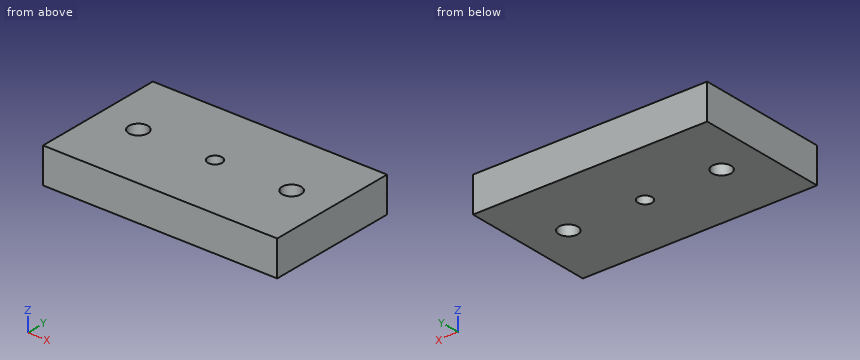
```python
from build123d import *

# Parameters (mm, degrees)
SKETCH1_W             = 40
SKETCH1_H             = 22.7
BOSS_EXTRUDE1_DEPTH   = 6
F_4_CLEARANCE_HOLE1_D = 3.2639
F_2_CLEARANCE_HOLE1_D = 2.4384


with BuildPart() as part:
    # Sketch1 → Boss-Extrude1 (new body)
    with BuildSketch(Plane.XY):
        Rectangle(SKETCH1_W, SKETCH1_H)
    extrude(amount=-BOSS_EXTRUDE1_DEPTH)

    # #4 Clearance Hole1 (through all)
    with Locations(Plane.XY):
        with Locations((-13.09, 0), (13.09, 0)):
            Hole(F_4_CLEARANCE_HOLE1_D / 2)

    # #2 Clearance Hole1 (through all)
    with Locations(Plane.XY):
        with Locations((0, 0)):
            Hole(F_2_CLEARANCE_HOLE1_D / 2)


solid = part.part
```
Check sheet for the modelled part. Datum: model origin and axes. Units: mm. Round coordinates to 2 decimals unless told otherwise and drop trailing zeros. Loops run counter-clockwise (first coordinate to the right, second up) from the corner with the lowest first, then second, coordinate; pieces in that order, holes last. Notation, with made-up numbers: (-28, 48.25) - (4, 48.25) arc R35 cw to (4, 82.25) - close; hole circle Ø2 at (-1.75, -9). An arc over 180 degrees is marked (long way). Answer as a JSON object with one key per item and string values. Group by question number.
Q1. Scan lines: line 1 along Y through (x, z) = (13.09, -1.8); line 2 along X through (y, z) = (-0.75, -0.4); line 3 along X through (y, z) = (1.25, -1.75). Record each from-to range of solid material in increasing order. Write a range as [from, to].
Q2. Sectioned sample at C-C, the plane z = -1.1. Enter the section's corners in (x, y).
Q3. Gauge pin test, flat ends, axial feed: P1, Ø2, axis at x = -13.09, y = 0, coming from the -Z side; P2, Ø5, axis at x = 13.09, y = 0, coming from the -Z side. Record the tip position at first contact, or that the pin passes through.
Q4. Sectioned sample at A-A, the plane x = -13.09. Enter the section's corners in (y, z).
Q5. Sectioned sample at B-B, the plane y = 0. Enter the section's corners in (x, z), plus the area to 3 significant figures.
Q6. Sectioned sample at D-D, the plane x = 0. Enter the section's corners in (y, z).
Solution:
{
 "1": {"line 1": "y = [-11.35, -1.63], [1.63, 11.35]", "line 2": "x = [-20, -14.54], [-11.64, -0.96], [0.96, 11.64], [14.54, 20]", "line 3": "x = [-20, -14.14], [-12.04, 12.04], [14.14, 20]"},
 "2": {"outline": "(-20, -11.35) - (20, -11.35) - (20, 11.35) - (-20, 11.35) - close; hole circle Ø3.26 at (-13.09, 0); hole circle Ø2.44 at (0, 0); hole circle Ø3.26 at (13.09, 0)"},
 "3": {"P1": "passes through", "P2": "stops at z = -6"},
 "4": {"outline": "(-11.35, -6) - (-1.63, -6) - (-1.63, 0) - (-11.35, 0) - close; (1.63, -6) - (11.35, -6) - (11.35, 0) - (1.63, 0) - close"},
 "5": {"outline": "(-20, -6) - (-14.72, -6) - (-14.72, 0) - (-20, 0) - close; (-11.46, -6) - (-1.22, -6) - (-1.22, 0) - (-11.46, 0) - close; (1.22, -6) - (11.46, -6) - (11.46, 0) - (1.22, 0) - close; (14.72, -6) - (20, -6) - (20, 0) - (14.72, 0) - close", "area": "186 mm²"},
 "6": {"outline": "(-11.35, -6) - (-1.22, -6) - (-1.22, 0) - (-11.35, 0) - close; (1.22, -6) - (11.35, -6) - (11.35, 0) - (1.22, 0) - close"}
}
